```python
from build123d import *

# Parameters (mm, degrees)
SKETCH1_R           = 3
SKETCH1_R_2         = 4.5
BOSS_EXTRUDE1_DEPTH = 5


with BuildPart() as part:
    # Sketch1 → Boss-Extrude1 (new body)
    # profile 1 of 3: a face of its own
    with BuildSketch(Plane.XY):
        with BuildLine():
            Line((-1.386138614, 6.861386139), (-25, 4.5))
            ThreePointArc((-25, 4.5), (-21.818019485, 3.181980515), (-20.5, 0))
            ThreePointArc((-20.5, 0), (-21.818019485, -3.181980515), (-25, -4.5))
            Line((-25, -4.5), (-1.386138614, -6.861386139))
            ThreePointArc((-1.386138614, -6.861386139), (-7, 0), (-1.386138614, 6.861386139))
        make_face()
    # profile 2 of 3: a face of its own
    with BuildSketch(Plane.XY):
        with BuildLine():
            Line((0, 7), (-1.386138614, 6.861386139))
            ThreePointArc((-1.386138614, 6.861386139), (-7, 0), (-1.386138614, -6.861386139))
            Line((-1.386138614, -6.861386139), (0, -7))
            ThreePointArc((0, -7), (4.949747468, -4.949747468), (7, 0))
            ThreePointArc((7, 0), (4.949747468, 4.949747468), (0, 7))
        make_face()
        Circle(SKETCH1_R, mode=Mode.SUBTRACT)
    # profile 3 of 3: a face of its own
    with BuildSketch(Plane.XY):
        with Locations((-25, 0)):
            Circle(SKETCH1_R_2)
        with Locations((-25, 0)):
            Circle(SKETCH1_R, mode=Mode.SUBTRACT)
    extrude(amount=BOSS_EXTRUDE1_DEPTH)


solid = part.part
```
Source: CAD feature listing. Evaluate the final solid. Frame: model axes, mm. Round coordinates to 2 decimals unless told otherwise and drop trailing zeros. Loops run counter-clockwise (first coordinate to the right, second up) from the corner with the lowest first, then second, coordinate; pieces in that order, holes last.
1. Mould query, pull axis X, two halves, no side actions, for faces 1 (the cylindrical face through (-29.5, 0.1, 2.5)), 2 (the flat face through (-12, 0, 0)), 3 (the cylindrical face through (-28, 0, 2)). Classes: released by +X, released by -X, zero draft, split by the parting line, or undercut.
2. Ray query, L1, parallel to Y at x = -25, z = 3.5; L2, parallel to X at y = 2.5, z = 2.8; L3, parallel to X at y = 1.75, z = 4.85. Return the intervals inside material, ascending.
3. Section query B-B on x = -2.5. Output: boundary loops of the cut face in (y, z), and give its area (3 significant figures).
4. Section query D-D on x = -16. Output: boundary loops of the cut face in (y, z), and give its area (3 significant figures).
5. Contact query for flat-ended pins moving along their axis: pin 1 (3 mm diameter, centred on y = 0.5, z = 2.5, fed in from -X); pin 2 (1.5 mm diameter, centred on x = 2, z = 4, fed in from +Y); pin 3 (3.5 mm diameter, centred on x = 0, y = 0, fed in from +Z). Output: stop coordinate, or through.
6. Section query A-A on z = 1.9. Output: boundary loops of the cut face in (x, y), and give its area (3 significant figures).
7. Section query C-C on y = 2.5. Output: boundary loops of the cut face in (x, z), and give its area (3 significant figures).
Answers below:
1. face 1: released by -X
1. face 2: zero draft
1. face 3: undercut
2. L1: y = -4.5 to -3, 3 to 4.5
2. L2: x = -28.74 to -26.66, -23.34 to -1.66, 1.66 to 6.54
2. L3: x = -29.15 to -27.44, -22.56 to -2.44, 2.44 to 6.78
3. outline: (-6.75, 0) - (-1.66, 0) - (-1.66, 5) - (-6.75, 5) - close; (1.66, 0) - (6.75, 0) - (6.75, 5) - (1.66, 5) - close
3. area: 50.9 mm2
4. outline: (-5.4, 0) - (5.4, 0) - (5.4, 5) - (-5.4, 5) - close
4. area: 54.0 mm2
5. pin 1: stops at x = -29.5
5. pin 2: stops at y = 6.89
5. pin 3: passes through
6. outline: (-25, -4.5) - (0, -7) arc R7 ccw to (0, 7) - (-25, 4.5) arc R4.5 ccw to start; hole circle Ø6 at (-25, 0); hole circle Ø6 at (0, 0)
6. area: 340 mm2
7. outline: (-28.74, 0) - (-26.66, 0) - (-26.66, 5) - (-28.74, 5) - close; (-23.34, 0) - (-1.66, 0) - (-1.66, 5) - (-23.34, 5) - close; (1.66, 0) - (6.54, 0) - (6.54, 5) - (1.66, 5) - close
7. area: 143 mm2
